Geometry: see drawing. Coordinates: mm, zero at the bounding-box minimum. Give positions to 0.01 mm unless a question says otherwise; leave off trailing zeros. Write each loop counter-clockwise with the first axis right and the second up, starting at its lowest first coordinate (ties: lowest second). Pieces come first, ordered by that corner, then holes. Notation, with made-up numbers: (69, 76.5) -> (109, 76.5) arc R30 ccw to (109, 114.5) -> close; hole circle Ø5 at (60.5, -8). An arc over 180 degrees is marked (long way). Write item = value, one per line.
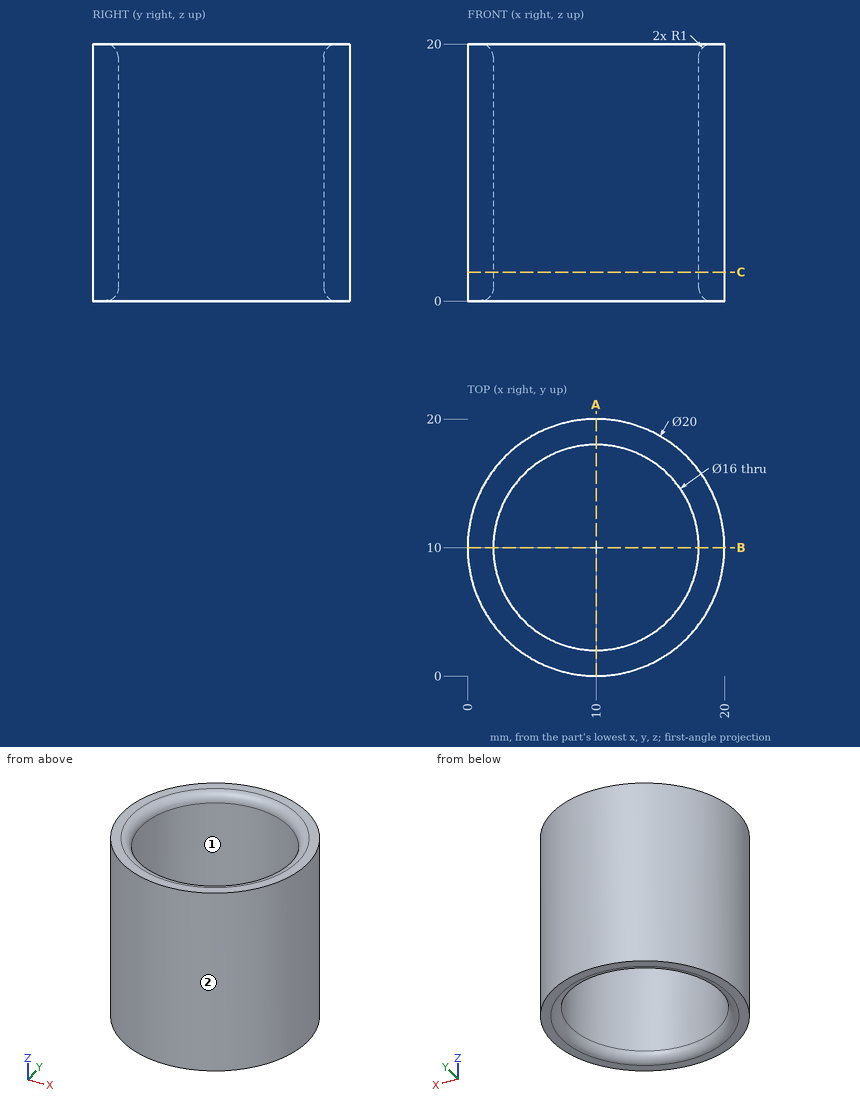
(1) Material intervals for line 1 (Y direction, x = 10, z = 4.75); line 2 (Y direction, x = 12.5, z = 4.75); line 3 (X direction, y = 14.25, z = 1), sorted ascending.
Values follow:
line_1 = 0 to 2, 18 to 20
line_2 = 0.32 to 2.4, 17.6 to 19.68
line_3 = 0.95 to 3.22, 16.78 to 19.05
(2) Section query C-C (z = 2.25). Return loops of the section in (x, y), plus the area to 3 significant figures.
Values follow:
outline = circle Ø20 at (10, 10); hole circle Ø16 at (10, 10)
area = 113 mm2
(3) Pull-direction query (X, two-part tool) for the marked faces 1 and 2; classes: pulls with the +X half, pulls with the -X half, needs draft (parallel to the pull), parting line crosses it, or undercut.
Values follow:
face_1 = undercut
face_2 = parting line crosses it
(4) Section query A-A (x = 10). Return loops of the section in (y, z), plus the area to 3 significant figures.
Values follow:
outline = (0, 0) -> (1, 0) arc R1 ccw to (2, 1) -> (2, 19) arc R1 ccw to (1, 20) -> (0, 20) -> close; (18, 1) arc R1 ccw to (19, 0) -> (20, 0) -> (20, 20) -> (19, 20) arc R1 ccw to (18, 19) -> close
area = 79.1 mm2
(5) First-contact query: pin 1 (2 mm diameter, centred on y = 3.5, z = 7, fed in from -X); pin 2 (3 mm diameter, centred on y = 13.5, z = 12, fed in from +X); pin 3 (1.5 mm diameter, centred on y = 15, z = 3, fed in from +X). Flat tips, straight axial feed; report the tip coordinate or a pass-through.
Values follow:
pin_1 = 1.65
pin_2 = 19.8
pin_3 = 19.05
